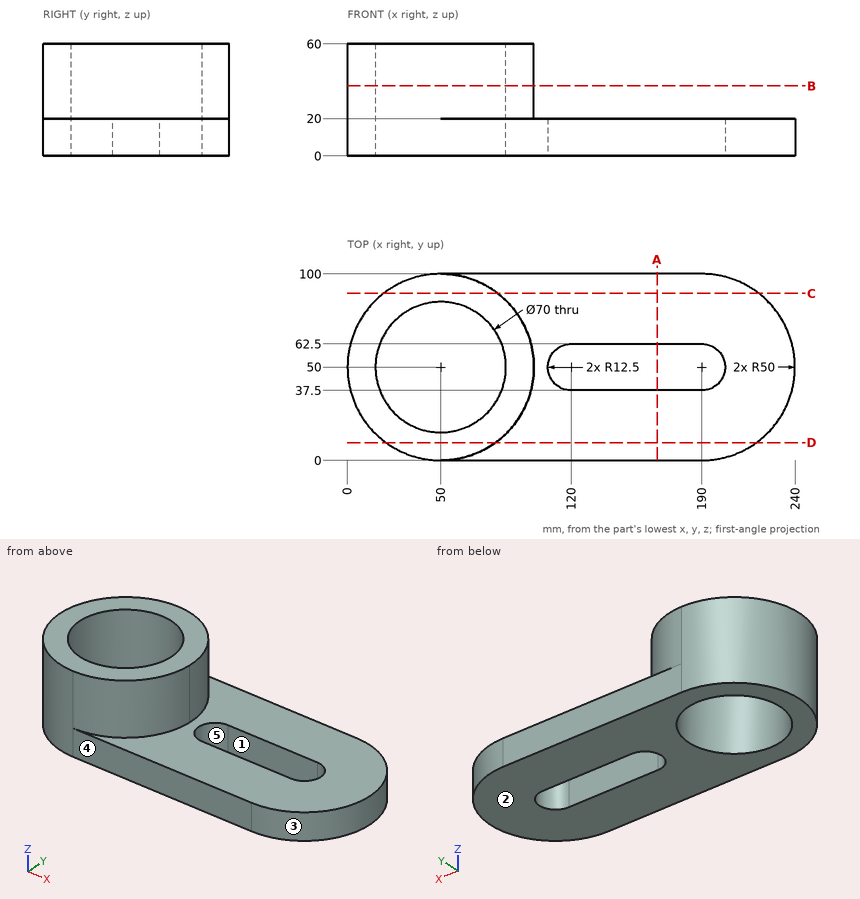
Answer from the drawing. Dimensions are ordinates in mm from the lowest x, y and z of the part. A direction names the side the tool comes from. Give positions to 0.01 mm unless a question says otherwise; leave off trailing zeros. Order: outer loops, then holes, each group sorted by start corner. A loop starts at its lowest first (then second) coordinate and runs counter-clockwise, first axis right, second up. Notation, with made-up numbers: (-10.5, 29.5) - (14.5, 29.5) arc R13 ccw to (14.5, 54.5) - close; hole circle Ø6 at (-13, 76). An arc over 180 degrees is marked (long way). One line per item, written item: value. Start each with the question number.
1. Which of the six approach directions +Z, -Z, +X, -X, +Y, -Y give full straight-line access (tool end or side, diameter ignored) to the marked faces 4 and 5?
2. Section C-C, the plane y = 89.5 is taken. Write down the section's boundary in (x, z).
3. Section A-A, the plane x = 166 is taken. Write down the section's boundary in (y, z), then the cut area to 3 significant figures.
4. Consider line 1 (Y direction, x = 158.5, z = 6); line 2 (Y direction, x = 50, z = 15); line 3 (Z direction, x = 194, y = 70.5). Determine where each line is inside the solid, lowest interval first.
5. For a pull along Y with two mould halves and no side action, classify the marked faces 1, 2 and 3 as released by +Y, released by -Y, zero draft, split by the parting line, or undercut.
6. Each of these flat-tipped pins is pushed along its axis until it touches: pin 1 Ø2 at (x, y) = (154.5, 83.5) entering from +Z; pin 2 Ø12 at (y, z) = (32, 11) entering from +X; pin 3 Ø6 at (y, z) = (87, 39.5) entering from +X. Where does it stop, or does it pass through?
7. Section B-B, the plane z = 37.5 is taken. Write down the section's boundary in (x, y).
8. Section D-D, the plane y = 9.5 is taken. Write down the section's boundary in (x, z), then the cut area to 3 significant figures.
Filled sheet:
1. face 4: +Z, -Z, +X, -X, -Y
1. face 5: +Z, -Z
2. outline: (19.34, 0) - (220.66, 0) - (220.66, 20) - (80.66, 20) - (80.66, 60) - (19.34, 60) - close
3. outline: (0, 0) - (37.5, 0) - (37.5, 20) - (0, 20) - close; (62.5, 0) - (100, 0) - (100, 20) - (62.5, 20) - close
3. area: 1,500 mm²
4. line 1: 0 to 37.5, 62.5 to 100
4. line 2: 0 to 15, 85 to 100
4. line 3: 0 to 20
5. face 1: undercut
5. face 2: zero draft
5. face 3: split by the parting line
6. pin 1: z = 20
6. pin 2: x = 238.54
6. pin 3: x = 86.66
7. outline: circle Ø100 at (50, 50); hole circle Ø70 at (50, 50)
8. outline: (20.68, 0) - (219.32, 0) - (219.32, 20) - (79.32, 20) - (79.32, 60) - (20.68, 60) - close
8. area: 6,320 mm²
